```python
from build123d import *

# Parameters (mm, degrees)
BASE_FLANGE1_DEPTH = 1613
CUT_EXTRUDE1_REACH = 1615.387
SKETCH6_R          = 4.5
FILLET1_R          = 3
CUT_EXTRUDE2_REACH = 1615.387
LPATTERN1_COUNT    = 4
LPATTERN1_PITCH    = 529
CUT_EXTRUDE3_REACH = 1615.198
SKETCH11_R         = 4.5
LPATTERN2_COUNT    = 3
LPATTERN2_PITCH    = 529
CUT_EXTRUDE4_REACH = 1615.198
SKETCH12_R         = 4.5


# Sheet-metal steps are written as plain solids
with BuildPart() as part:
    # Sketch1 → Base-Flange1 (new body)
    with BuildSketch(Plane(origin=(0, 0, 0), x_dir=(1, 0, 0), z_dir=(0, 1, 0))):
        with BuildLine():
            Line((-12.5, -25), (-12.5, -4.5))
            ThreePointArc((-12.5, -4.5), (-11.181980515, -1.318019485), (-8, 0))
            Line((-8, 0), (8, 0))
            ThreePointArc((8, 0), (11.181980515, -1.318019485), (12.5, -4.5))
            Line((12.5, -4.5), (12.5, -25))
            Line((12.5, -25), (9.5, -25))
            Line((9.5, -25), (9.5, -4.5))
            ThreePointArc((9.5, -4.5), (9.060660172, -3.439339828), (8, -3))
            Line((8, -3), (-8, -3))
            ThreePointArc((-8, -3), (-9.060660172, -3.439339828), (-9.5, -4.5))
            Line((-9.5, -4.5), (-9.5, -25))
            Line((-9.5, -25), (-12.5, -25))
        make_face()
    extrude(amount=BASE_FLANGE1_DEPTH)

    # Sketch6 → Cut-Extrude1 (cut, up to next)
    with BuildSketch(Plane.ZY.offset(12.5), mode=Mode.PRIVATE) as cut_extrude1_sk1:
        with Locations((15.5, 13)):
            Circle(SKETCH6_R)
    cut_extrude1_tool1 = extrude(cut_extrude1_sk1.sketch, amount=-CUT_EXTRUDE1_REACH, mode=Mode.PRIVATE) & part.part
    cut_extrude1 = cut_extrude1_tool1.solids().sort_by_distance((-12.5, 13, 15.5))[0]
    add(cut_extrude1, mode=Mode.SUBTRACT)

    # Fillet1
    fillet1_edges = [part.edges().sort_by_distance(p)[0] for p in [
        (11, 0, 25),
        (-11, 0, 25),
        (11, 1613, 25),
        (-11, 1613, 25),
    ]]
    fillet(fillet1_edges, radius=FILLET1_R)

    # Sketch7 → Cut-Extrude2 (cut, up to next)
    with BuildSketch(Plane(origin=(12.5, 0, 0), x_dir=(0, 0, -1), z_dir=(1, 0, 0)), mode=Mode.PRIVATE) as cut_extrude2_sk1:
        with BuildLine():
            Line((-18.5, 18), (-12.5, 18))
            ThreePointArc((-12.5, 18), (-7.5, 13), (-12.5, 8))
            Line((-12.5, 8), (-18.5, 8))
            ThreePointArc((-18.5, 8), (-23.5, 13), (-18.5, 18))
        make_face()
    cut_extrude2_tool1 = extrude(cut_extrude2_sk1.sketch, amount=-CUT_EXTRUDE2_REACH, mode=Mode.PRIVATE) & part.part
    cut_extrude2 = cut_extrude2_tool1.solids().sort_by_distance((12.5, 13, 15.5))[0]
    add(cut_extrude2, mode=Mode.SUBTRACT)

    # LPattern1: Cut-Extrude1, Cut-Extrude2 ×4
    with Locations(*[(0, i * LPATTERN1_PITCH, 0) for i in range(1, LPATTERN1_COUNT)]):
        add(cut_extrude1, mode=Mode.SUBTRACT)
        add(cut_extrude2, mode=Mode.SUBTRACT)

    # Sketch11 → Cut-Extrude3 (cut, up to next)
    with BuildSketch(Plane.XY.offset(3), mode=Mode.PRIVATE) as cut_extrude3_sk1:
        with Locations((0, 25)):
            Circle(SKETCH11_R)
    cut_extrude3_tool1 = extrude(cut_extrude3_sk1.sketch, amount=-CUT_EXTRUDE3_REACH, mode=Mode.PRIVATE) & part.part
    cut_extrude3 = cut_extrude3_tool1.solids().sort_by_distance((0, 25, 3))[0]
    add(cut_extrude3, mode=Mode.SUBTRACT)

    # LPattern2: Cut-Extrude3 ×3
    with Locations(*[(0, i * LPATTERN2_PITCH, 0) for i in range(1, LPATTERN2_COUNT)]):
        add(cut_extrude3, mode=Mode.SUBTRACT)

    # Sketch12 → Cut-Extrude4 (cut, up to next)
    with BuildSketch(Plane.XY.offset(3), mode=Mode.PRIVATE) as cut_extrude4_sk1:
        with Locations((0, 1588)):
            Circle(SKETCH12_R)
    cut_extrude4_tool1 = extrude(cut_extrude4_sk1.sketch, amount=-CUT_EXTRUDE4_REACH, mode=Mode.PRIVATE) & part.part
    add(cut_extrude4_tool1.solids().sort_by_distance((0, 1588, 3))[0], mode=Mode.SUBTRACT)


solid = part.part
```
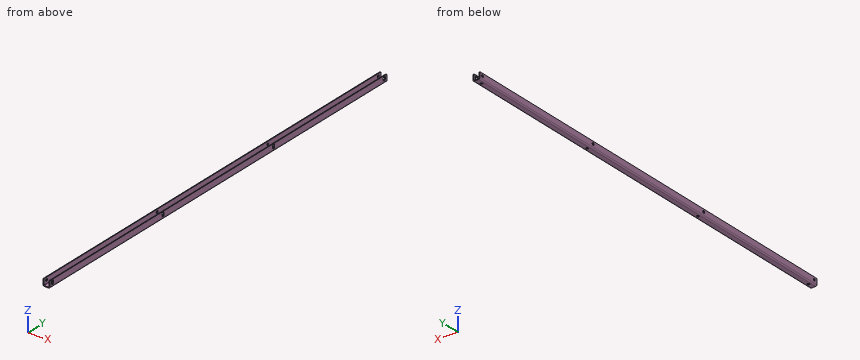
Geometry check sheet. Reference: the model listing, model coordinates, mm. Round coordinates to 2 decimals unless told otherwise and drop trailing zeros. Order: outer loops, then holes, each group sorted by start corner. A loop starts at its lowest first (then second) coordinate and runs counter-clockwise, first axis right, second up. Notation, with made-up numbers: (48, 38.5) -> (74, 38.5) arc R28 cw to (74, 66.5) -> close; hole circle Ø2 at (85, -36). An arc over 180 degrees is marked (long way). Return JSON: item names as keys, results as strings. Group by question number.
Q1. Gauge pin test, flat ends, axial feed: pin 1 (6 mm diameter, centred on x = -4.5, z = 4, fed in from -Y); pin 2 (2 mm diameter, centred on x = -8, z = 12.5, fed in from -Y); pin 3 (6 mm diameter, centred on x = -3, y = 361, fed in from +Z). Record the tip position at first contact, or that the pin passes through.
Q2. Section check A-A, the plane y = 385. Record the boundary of the cut face in (x, z).
Q3. Material ranges on probe 1 along Y at (x, z) = (0, 1.25); probe 2 along Y at (x, z) = (11, 19.75); probe 3 along X at (y, z) = (572, 3.75), recorded low to high. Write a range as from..to.
Numbers:
{
 "1": {"pin 1": "y = 0", "pin 2": "through", "pin 3": "z = 3"},
 "2": {"outline": "(-12.5, 4.5) arc R4.5 ccw to (-8, 0) -> (8, 0) arc R4.5 ccw to (12.5, 4.5) -> (12.5, 25) -> (9.5, 25) -> (9.5, 4.5) arc R1.5 cw to (8, 3) -> (-8, 3) arc R1.5 cw to (-9.5, 4.5) -> (-9.5, 25) -> (-12.5, 25) -> close"},
 "3": {"probe 1": "0..20.5, 29.5..549.5, 558.5..1078.5, 1087.5..1583.5, 1592.5..1613", "probe 2": "0..8.16, 17.84..537.16, 546.84..1066.16, 1075.84..1595.16, 1604.84..1613", "probe 3": "-12.44..-9.3, 9.3..12.44"}
}
